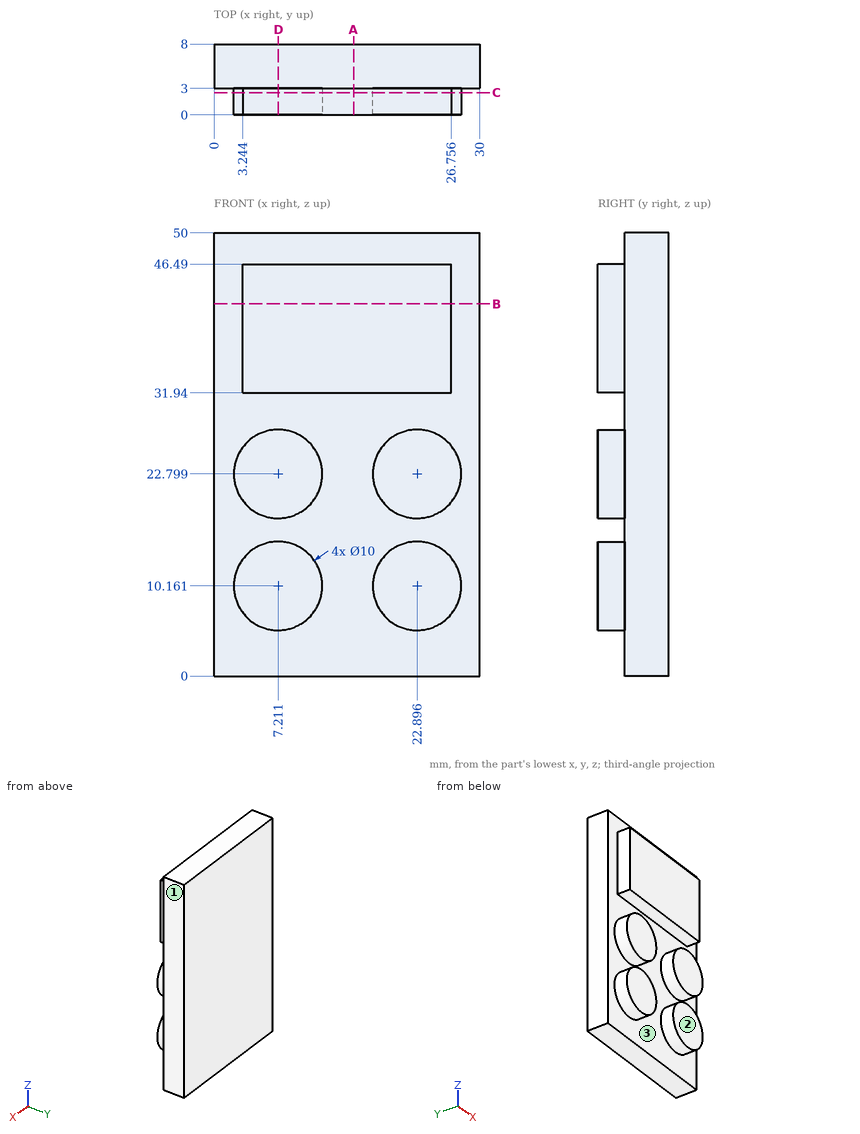
Here's the drawing with two shaded views (mm, measured from the low corner). I have some questions. Round coordinates to 2 decimals unless told otherwise and drop trailing zeros. Write each loop counter-clockwise with the first axis right and the second up, starting at its lowest first coordinate (ties: lowest second). Pieces come first, ordered by that corner, then holes.
(1) Thinking about a two-plate mould opening in X: for the marked faces 1, 2 and 3, which applies, +X half, -X half, draft (parallel to the pull), parting line (faces both ways), or undercut?
Findings below:
face 1: +X half
face 2: draft
face 3: undercut
(2) If I drill on probe 1 along Z at (x, y) = (18.75, 0.5) (1 decimal); probe 2 along Y at (x, z) = (12.25, 5.5); probe 3 along Z at (x, y) = (19.75, 1) (1 decimal), over which ranges is the centre line in solid material (lowest first)?
Findings below:
probe 1: z = 7.4 to 13, 20 to 25.6, 31.9 to 46.5
probe 2: y = 3 to 8
probe 3: z = 6.3 to 14, 18.9 to 26.7, 31.9 to 46.5
(3) Suppose I cut it at C-C on y = 2.5. Write out the boundary of the cut face in (x, z) (1 decimal).
Findings below:
outline: circle Ø10 at (7.2, 10.2); circle Ø10 at (7.2, 22.8); (3.2, 31.9) - (26.8, 31.9) - (26.8, 46.5) - (3.2, 46.5) - close; circle Ø10 at (22.9, 10.2); circle Ø10 at (22.9, 22.8)
(4) Suppose I cut it at B-B on z = 42. Write out the boundary of the cut face in (x, y) (1 decimal).
Findings below:
outline: (0, 3) - (3.2, 3) - (3.2, 0) - (26.8, 0) - (26.8, 3) - (30, 3) - (30, 8) - (0, 8) - close
(5) For pin 1 (0.9 mm diameter, centred on x = 19.5, y = 1.5, fed in from -Z); pin 2 (1.5 mm diameter, centred on y = 2, z = 40, fed in from +X); pin 3 (1.5 mm diameter, centred on x = 20.5, y = 2, fed in from +Z), each with a flat end and sliding along its axis, tell me the tip position at first contact or that it passes through.
Findings below:
pin 1: stops at z = 6.12
pin 2: stops at x = 26.76
pin 3: stops at z = 46.49
(6) Suppose I cut it at D-D on x = 7.25. Write out the boundary of the cut face in (y, z), and give its area (3 significant figures).
Findings below:
outline: (0, 5.16) - (3, 5.16) - (3, 0) - (8, 0) - (8, 50) - (3, 50) - (3, 46.49) - (0, 46.49) - (0, 31.94) - (3, 31.94) - (3, 27.8) - (0, 27.8) - (0, 17.8) - (3, 17.8) - (3, 15.16) - (0, 15.16) - close
area: 354 mm2
(7) Suppose I cut it at A-A on x = 15.75. Write out the boundary of the cut face in (y, z).
Findings below:
outline: (0, 31.94) - (3, 31.94) - (3, 0) - (8, 0) - (8, 50) - (3, 50) - (3, 46.49) - (0, 46.49) - close
